Autodesk Fusion 360 part; units mm, degrees
sketch "Sketch1" plane through (0, 0, 0) normal (0, 0, 1) x (1, 0, 0)
  circle A0 centre (27.5702, 32.2128) radius 2
  circle A1 centre (27.5702, 17.2128) radius 2
  circle A2 centre (83.5354, 17.2128) radius 2
  circle A3 centre (83.5354, 32.2128) radius 2
  line L0 (14.5612, 17.2128) -> (18.5612, 17.2128)
  line L1 (18.5612, 17.2128) -> (18.5612, 32.2128)
  line L2 (18.5612, 32.2128) -> (14.5612, 32.2128)
  line L3 (96.5612, 17.2128) -> (92.5612, 17.2128)
  line L4 (92.5612, 17.2128) -> (92.5612, 32.2128)
  line L5 (92.5612, 32.2128) -> (96.5612, 32.2128)
  line L6 (14.5612, 32.2128) -> (14.5612, 34.134)
  line L7 (14.5612, 34.134) -> (14.5612, 47.2128)
  line L8 (14.5612, 17.2128) -> (14.5612, -12.7872)
  line L9 (96.5612, -12.7872) -> (96.5612, 4.1678)
  line L10 (96.5612, 4.1678) -> (96.5612, 17.2128)
  line L11 (96.5612, 32.2128) -> (96.5612, 47.2128)
  line L12 (47.5702, 37.2128) -> (63.5354, 37.2128)
  line L13 (63.5354, 37.2128) -> (63.5354, 47.2128)
  line L14 (47.5702, 47.2128) -> (47.5702, 37.2128)
  line L15 (63.5354, 12.2128) -> (47.5702, 12.2128)
  line L16 (47.5702, 12.2128) -> (47.5702, -12.7872)
  line L17 (63.5354, -12.7872) -> (63.5354, 12.2128)
  line L18 (96.5612, -12.7872) -> (63.5354, -12.7872)
  line L19 (47.5702, -12.7872) -> (14.5612, -12.7872)
  line L20 (39.5612, 47.2128) -> (39.5612, 43.2128)
  line L21 (39.5612, 43.2128) -> (24.5612, 43.2128)
  line L22 (24.5612, 43.2128) -> (24.5612, 47.2128)
  line L23 (86.5612, 47.2128) -> (86.5612, 43.2128)
  line L24 (86.5612, 43.2128) -> (71.5444, 43.2128)
  line L25 (71.5444, 43.2128) -> (71.5444, 47.2128)
  line L26 (24.5612, 47.2128) -> (14.5612, 47.2128)
  line L27 (39.5612, 47.2128) -> (47.5702, 47.2128)
  line L28 (63.5354, 47.2128) -> (71.5444, 47.2128)
  line L29 (86.5612, 47.2128) -> (96.5612, 47.2128)
  dimension "d45" = 30
  dimension "d46" = 30
extrude "Extrude9" add sketch "Sketch1" along normal blind 4
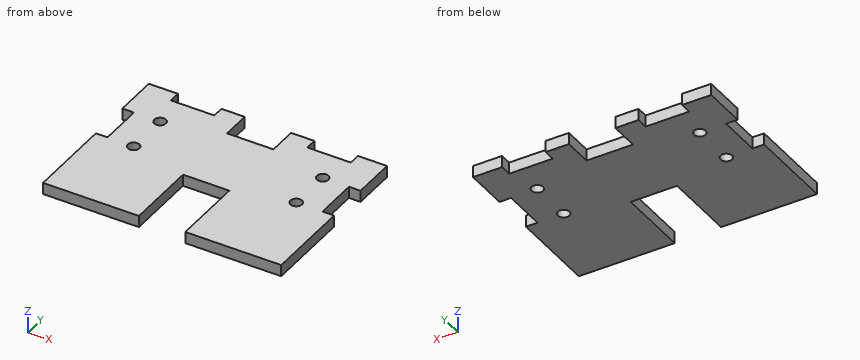
The model under review builds one solid part; all positions refer to its coordinate system, in mm. Coordinates: 2 decimals unless noted, no trailing zeros. Order: outer loops, then holes, each group sorted by start corner. A loop starts at its lowest first (then second) coordinate and runs counter-clockwise, first axis right, second up. Notation, with made-up numbers: (56, 81) -> (80, 81) arc R21 ccw to (80, 85) -> close; hole circle Ø7 at (22, -9.75). An arc over 180 degrees is marked (long way). Answer in a Markdown table with one row per item. Add a question column.
Item 1: We need section C-C on y = 28. Write out the cut boundary in (x, z), plus the area to 3 significant figures.
Item 2: We need section B-B on x = 74.5. Write out the cut boundary in (y, z), plus the area to 3 significant figures.
Item 3: Clearance check with flat-ended pins moving along their axes: pin 1 (1 mm diameter, centred on y = 19, z = 3, fed in from +X); pin 2 (3 mm diameter, centred on x = 83.54, y = 32.21, fed in from +Z); pin 3 (1.2 mm diameter, centred on x = 55.5, z = 1, fed in from +Y). State where each tip first meets the part, or that it passes through.
Item 4: We need section A-A on z = 2.75. Give the number of separate pieces and of enclosed holes in the cut face, plus the area to 3 significant figures.
Item 5: To check wall thickness, follow probe 1 along X at (y, z) = (44.5, 3.8); probe 2 along X at (y, z) = (-4, 3.05); probe 3 along Y at (x, z) = (86.5, 0.45). State the ranges of each line that lie inside material, in increasing order.
Final values:
| question | item | result |
|---|---|---|
| 1 | outline | (18.56, 0) -> (92.56, 0) -> (92.56, 4) -> (18.56, 4) -> close |
| 1 | area | 296 mm2 |
| 2 | outline | (-12.79, 0) -> (43.21, 0) -> (43.21, 4) -> (-12.79, 4) -> close |
| 2 | area | 224 mm2 |
| 3 | pin 1 | stops at x = 92.56 |
| 3 | pin 2 | passes through |
| 3 | pin 3 | stops at y = 37.21 |
| 4 | separate pieces | 1 |
| 4 | enclosed holes | 4 |
| 4 | area | 4,070 mm2 |
| 5 | probe 1 | x = 14.56 to 24.56, 39.56 to 47.57, 63.54 to 71.54, 86.56 to 96.56 |
| 5 | probe 2 | x = 14.56 to 47.57, 63.54 to 96.56 |
| 5 | probe 3 | y = -12.79 to 43.21 |
